```python
from build123d import *

# Parameters (mm, degrees)
BOSS_EXTRUDE1_DEPTH = 8
SKETCH2_R           = 8
CUT_EXTRUDE1_DEPTH  = 5
SKETCH3_R           = 3.5
CUT_EXTRUDE2_DEPTH  = 164.176285042
SKETCH4_R           = 8
CUT_EXTRUDE3_DEPTH  = 5
SKETCH5_R           = 3.5
CUT_EXTRUDE4_DEPTH  = 164.176285042


with BuildPart() as part:
    # Sketch1 → Boss-Extrude1 (new body)
    with BuildSketch(Plane(origin=(0, 0, 0), x_dir=(1, 0, 0), z_dir=(0, 1, 0))):
        with BuildLine():
            Line((-12.5, 0), (-12.5, -150))
            ThreePointArc((-12.5, -150), (0, -162.5), (12.5, -150))
            Line((12.5, -150), (12.5, 0))
            ThreePointArc((12.5, 0), (0, 12.5), (-12.5, 0))
        make_face()
    extrude(amount=BOSS_EXTRUDE1_DEPTH)

    # Sketch2 → Cut-Extrude1 (cut)
    with BuildSketch(Plane(origin=(0, 8, 0), x_dir=(1, 0, 0), z_dir=(0, 1, 0))):
        with Locations(Location((0, 0, 0), (0, 0, 270))):
            Circle(SKETCH2_R)
    extrude(amount=-CUT_EXTRUDE1_DEPTH, mode=Mode.SUBTRACT)

    # Sketch3 → Cut-Extrude2 (cut, through all)
    with BuildSketch(Plane(origin=(0, 8, 0), x_dir=(1, 0, 0), z_dir=(0, 1, 0))):
        with Locations(Location((0, 0, 0), (0, 0, 270))):
            Circle(SKETCH3_R)
    extrude(amount=-CUT_EXTRUDE2_DEPTH, mode=Mode.SUBTRACT)

    # Sketch4 → Cut-Extrude3 (cut)
    with BuildSketch(Plane(origin=(0, 8, 0), x_dir=(1, 0, 0), z_dir=(0, 1, 0))):
        with Locations(Location((0, -150, 0), (0, 0, 270))):
            Circle(SKETCH4_R)
    extrude(amount=-CUT_EXTRUDE3_DEPTH, mode=Mode.SUBTRACT)

    # Sketch5 → Cut-Extrude4 (cut, through all)
    with BuildSketch(Plane(origin=(0, 8, 0), x_dir=(1, 0, 0), z_dir=(0, 1, 0))):
        with Locations(Location((0, -150, 0), (0, 0, 270))):
            Circle(SKETCH5_R)
    extrude(amount=-CUT_EXTRUDE4_DEPTH, mode=Mode.SUBTRACT)


solid = part.part
```
Can you work these out from the model? Positions are in its coordinate system, mm. A direction names the side the tool comes from. Coordinates: 2 decimals unless noted, no trailing zeros. Write each loop counter-clockwise with the first axis right and the second up, starting at its lowest first coordinate (ties: lowest second). Pieces come first, ordered by that corner, then holes. Notation, with made-up numbers: M 34.5,88.25 L 39.5,88.25 A21 ccw 39.5,100.25 Z; hole C 55.25,53 d4. An arc over 180 degrees is marked long. Write item = value, one per line. Start each with the question number.
Q1. If we section it at C-C, the plane x = 10.5: Write out the boundary of the cut face in (y, z).
Q2. If we section it at B-B, the plane y = 1.75: Write out the boundary of the cut face in (x, z).
Q3. On a 3-axis mill with a long thin cutter (end or side, diameter ignored), from which of +Z, -Z, +X, -X, +Y, -Y can I reach the whole of each face in a straight line? I mean faces 4 (the face through (0, 6, 142)), 5 (the face through (12.5, 4, 76)). Say none if no direction works.
Q4. Thinking about a two-plate mould opening in Z: for faces 1 (the face through (-12.5, 4, 74)), 2 (the face through (-7.81, 5.54, -1.73)), 3 (the face through (0.275, 3.944, -12.497)), which applies, released by +Z, released by -Z, zero draft, split by the parting line, or undercut?
Q5. If I drill on L1, parallel to X at y = 1.15, z = 150; L2, parallel to Z at x = -6.25, y = 4; L3, parallel to X at y = 4.05, z = 150, over which ranges is the centre line in solid material (lowest first)? Write a range as [from, to].
Q6. If we section it at A-A, the plane x = 0: Write out the boundary of the cut face in (y, z).
Q7. I'm going to push flat-ended pins straight in: pin 1 (13 mm diameter, centred on x = 0, z = 150, fed in from +Y); pin 2 (1.5 mm diameter, centred on x = -4, y = 4, fed in from +Z). Where does each tip first touch, or does it pass through?
Check sheet entries:
q1.outline = M 0,-6.78 L 8,-6.78 L 8,156.78 L 0,156.78 Z
q2.outline = M -12.5,0 A12.5 ccw 12.5,0 L 12.5,150 A12.5 ccw -12.5,150 Z; hole C 0,0 d7; hole C 0,150 d7
q3.face_4 = +Y
q3.face_5 = +Z, -Z, +X, +Y, -Y
q4.face_1 = zero draft
q4.face_2 = undercut
q4.face_3 = released by -Z
q5.L1 = [-12.5, -3.5], [3.5, 12.5]
q5.L2 = [-10.83, -4.99], [4.99, 145.01], [154.99, 160.83]
q5.L3 = [-12.5, -8], [8, 12.5]
q6.outline = M 0,-12.5 L 8,-12.5 L 8,-8 L 3,-8 L 3,-3.5 L 0,-3.5 Z; M 0,3.5 L 3,3.5 L 3,8 L 8,8 L 8,142 L 3,142 L 3,146.5 L 0,146.5 Z; M 0,153.5 L 3,153.5 L 3,158 L 8,158 L 8,162.5 L 0,162.5 Z
q7.pin_1 = 3
q7.pin_2 = 162.07
